Verification items for the finished model (mm, model axes). Face numbers are marked on the shaded views. A direction names the side the tool comes from. Coordinates: 2 decimals unless noted, no trailing zeros. Write each loop counter-clockwise with the first axis right and the second up, starting at its lowest first coordinate (ties: lowest second). Pieces come first, ordered by that corner, then holes. Notation, with made-up numbers: (-3.5, 89) -> (30.5, 89) arc R12 cw to (30.5, 93) -> close; hole circle Ø6 at (47, -33). An arc over 180 degrees is marked (long way). Use CSV: the item, a comma, the result in double quotes.
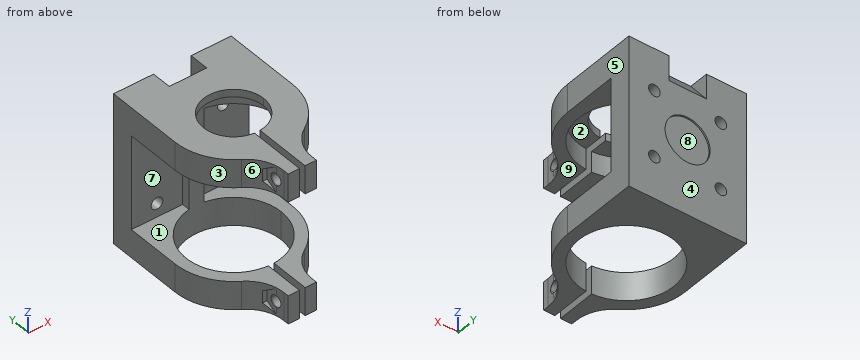
```python
from build123d import *

# Parameters (mm, degrees)
BOSS_EXTRUDE1_DEPTH   = 20
SKETCH2_W             = 3
SKETCH2_H             = 10.5
BOSS_EXTRUDE2_DEPTH   = 20
SKETCH4_W             = 31.3
SKETCH4_H             = 40
BOSS_EXTRUDE3_DEPTH   = 5
SKETCH5_W             = 25
SKETCH5_H             = 37.777747226
CUT_EXTRUDE2_DEPTH    = 13.65
SKETCH6_R             = 1.55
MOTORMOUNTHOLES_DEPTH = 6
CLAMPHOLES_REACH      = 38.211
SKETCH8_R             = 1.55
ENDSTOPPER_DEPTH      = 2
CUT_EXTRUDE7_START    = -15.65
SKETCH10_W            = 25
SKETCH10_H            = 37.777747226
CUT_EXTRUDE7_DEPTH    = 13.65
SKETCH11_W            = 25
SKETCH11_H            = 10.636850541
CUT_EXTRUDE8_DEPTH    = 4
FILLET1_START         = -20
FILLET1_DEPTH         = 2.1999999
FILLET1_START_2       = -14.6999999
FILLET1_2_DEPTH       = 2.1999999
FILLET1_START_3       = 12.5
FILLET1_3_DEPTH       = 2.1999999
FILLET1_START_4       = 17.8000001
FILLET1_4_DEPTH       = 2.1999999
FILLET1_START_5       = -17.8000001
FILLET1_5_DEPTH       = 3.1000002
FILLET1_START_6       = 14.6999999
FILLET1_6_DEPTH       = 3.1000002
FILLET1_START_7       = -8.389376218
FILLET1_7_OUTLINE_R   = 1.55
FILLET1_7_DEPTH       = 16.778752436
SKETCH13_W            = 10
SKETCH13_H            = 10
CUT_EXTRUDE10_REACH   = 40.348
CUT_EXTRUDE10_START   = 4
SKETCH15_R            = 3
CUT_EXTRUDE11_START   = -4
CUT_EXTRUDE11_DEPTH   = 3
SKETCH17_R            = 6
SHAFT_CLEARANCE_DEPTH = 0.4


with BuildPart() as part:
    # Sketch1 → Boss-Extrude1 (new, symmetric)
    with BuildSketch(Plane.XY):
        with BuildLine():
            Line((-15.65, 15.65), (-15.65, 0))
            ThreePointArc((-15.65, 0), (-11.066221106, 11.066221145), (5.4e-08, 15.65))
            Line((5.4e-08, 15.65), (-15.65, 15.65))
        make_face()
        with BuildLine():
            Line((15.65, 15.65), (5.4e-08, 15.65))
            ThreePointArc((5.4e-08, 15.65), (11.066221145, 11.066221106), (15.65, 0))
            Line((15.65, 0), (15.65, 15.65))
        make_face()
        with BuildLine():
            ThreePointArc((5.4e-08, 15.65), (-11.066221106, 11.066221145), (-15.65, 0))
            ThreePointArc((-15.65, 0), (-11.328283189, -10.797800702), (-0.75, -15.632018424))
            Line((-0.75, -15.632018424), (-0.75, -12.627747226))
            ThreePointArc((-0.75, -12.627747226), (-8.675684411, 9.206247878), (12.65, 0))
            ThreePointArc((12.65, 0), (9.206247878, -8.675684411), (0.75, -12.627747226))
            Line((0.75, -12.627747226), (0.75, -15.632018424))
            ThreePointArc((0.75, -15.632018424), (11.328283189, -10.797800702), (15.65, 0))
            ThreePointArc((15.65, 0), (11.066221145, 11.066221106), (5.4e-08, 15.65))
        make_face()
    extrude(amount=BOSS_EXTRUDE1_DEPTH, both=True)

    # Sketch2 → Boss-Extrude2 (add, symmetric)
    with BuildSketch(Plane.XY):
        with Locations((-2.25, -17.877747226)):
            Rectangle(SKETCH2_W, SKETCH2_H)
        with Locations((2.25, -17.877747226)):
            Rectangle(SKETCH2_W, SKETCH2_H)
    extrude(amount=BOSS_EXTRUDE2_DEPTH, both=True)

    # Sketch4 → Boss-Extrude3 (add)
    with BuildSketch(Plane(origin=(0, 15.65, 0), x_dir=(1, 0, 0), z_dir=(0, 1, 0))):
        Rectangle(SKETCH4_W, SKETCH4_H)
    extrude(amount=BOSS_EXTRUDE3_DEPTH)

    # Sketch5 → Cut-Extrude2 (cut)
    with BuildSketch(Plane(origin=(15.65, 0, 0), x_dir=(0, 0, -1), z_dir=(1, 0, 0))):
        with Locations((0, -4.238873613)):
            Rectangle(SKETCH5_W, SKETCH5_H)
    extrude(amount=-CUT_EXTRUDE2_DEPTH, mode=Mode.SUBTRACT)

    # Sketch6 → MotorMountHoles (cut)
    with BuildSketch(Plane(origin=(0, 20.65, 0), x_dir=(1, 0, 0), z_dir=(0, 1, 0))):
        with Locations(Location((-8.838834765, 8.838834765, 0), (0, 0, 270))):
            Circle(SKETCH6_R)
        with Locations(Location((8.838834765, 8.838834765, 0), (0, 0, 270))):
            Circle(SKETCH6_R)
        with Locations(Location((8.838834765, -8.838834765, 0), (0, 0, 270))):
            Circle(SKETCH6_R)
        with Locations(Location((-8.838834765, -8.838834765, 0), (0, 0, 270))):
            Circle(SKETCH6_R)
    extrude(amount=-MOTORMOUNTHOLES_DEPTH, mode=Mode.SUBTRACT)

    # ClampHoles: up to this face of the body (flat: up to its plane)
    clampholes_end = Plane(part.part.faces().sort_by_distance((3.75, -19.16091251, 16.25))[0])
    # Sketch8 → ClampHoles (cut, up to the picked face)
    with BuildSketch(Plane.ZY.offset(3.75), mode=Mode.PRIVATE) as clampholes_sk1:
        with Locations(Location((16.25, -19.194077794, 0), (0, 0, 270))):
            Circle(SKETCH8_R)
    clampholes_tool1 = split(extrude(clampholes_sk1.sketch, amount=-CLAMPHOLES_REACH, mode=Mode.PRIVATE), bisect_by=clampholes_end, keep=Keep.BOTH, mode=Mode.PRIVATE)
    # Sketch8 → ClampHoles (cut, up to the picked face)
    with BuildSketch(Plane.ZY.offset(3.75), mode=Mode.PRIVATE) as clampholes_sk2:
        with Locations(Location((-16.25, -19.194077794, 0), (0, 0, 270))):
            Circle(SKETCH8_R)
    clampholes_tool2 = split(extrude(clampholes_sk2.sketch, amount=-CLAMPHOLES_REACH, mode=Mode.PRIVATE), bisect_by=clampholes_end, keep=Keep.BOTH, mode=Mode.PRIVATE)
    add(clampholes_tool1.solids().sort_by(Axis((-3.75, -19.194078, 16.25), (1, 0, 0)))[0], mode=Mode.SUBTRACT)
    add(clampholes_tool2.solids().sort_by(Axis((-3.75, -19.194078, -16.25), (1, 0, 0)))[0], mode=Mode.SUBTRACT)

    # Sketch9 → EndStopper (add)
    with BuildSketch(Plane.XY.offset(20)):
        with BuildLine():
            ThreePointArc((12.65, 0), (-8.675684411, 9.206247878), (-0.75, -12.627747226))
            Line((-0.75, -12.627747226), (-0.75, -7.964766161))
            ThreePointArc((-0.75, -7.964766161), (-5.385164807, 5.916079783), (8, 0))
            ThreePointArc((8, 0), (5.916079783, -5.385164807), (0.75, -7.964766161))
            Line((0.75, -7.964766161), (0.75, -12.627747226))
            ThreePointArc((0.75, -12.627747226), (9.206247878, -8.675684411), (12.65, 0))
        make_face()
    extrude(amount=-ENDSTOPPER_DEPTH)

    # Sketch10 → Cut-Extrude7 (cut)
    with BuildSketch(Plane(origin=(0, 0, 0), x_dir=(0, 0, -1), z_dir=(1, 0, 0)).offset(CUT_EXTRUDE7_START)):
        with Locations((0, -4.238873613)):
            Rectangle(SKETCH10_W, SKETCH10_H)
    extrude(amount=CUT_EXTRUDE7_DEPTH, mode=Mode.SUBTRACT)

    # Sketch11 → Cut-Extrude8 (cut)
    with BuildSketch(Plane.ZY.offset(2)):
        with Locations((0, -17.809321955)):
            Rectangle(SKETCH11_W, SKETCH11_H)
    extrude(amount=-CUT_EXTRUDE8_DEPTH, mode=Mode.SUBTRACT)

    # Fillet1: read off the stored shape, not the designer's step
    # Fillet1 outline → Fillet1 (add)
    with BuildSketch(Plane.XY.offset(FILLET1_START)):
        with BuildLine():
            Line((3.75, -15.194077794), (3.75, -21.653175287))
            ThreePointArc((3.75, -21.653175287), (4.986261134, -16.83686123), (8.389376218, -13.211391549))
            ThreePointArc((8.389376218, -13.211391549), (6.150111782, -14.39092162), (3.75, -15.194077794))
        make_face()
        with BuildLine():
            ThreePointArc((-3.75, -15.194077794), (-6.150111782, -14.39092162), (-8.389376218, -13.21139155))
            ThreePointArc((-8.389376218, -13.21139155), (-4.986261134, -16.83686123), (-3.75, -21.653175287))
            Line((-3.75, -21.653175287), (-3.75, -15.194077794))
        make_face()
    extrude(amount=FILLET1_DEPTH)

    # Fillet1 2 outline → Fillet1 2 (add)
    with BuildSketch(Plane.XY.offset(FILLET1_START_2)):
        with BuildLine():
            Line((3.75, -15.194077794), (3.75, -21.653175287))
            ThreePointArc((3.75, -21.653175287), (4.986261134, -16.83686123), (8.389376218, -13.211391549))
            ThreePointArc((8.389376218, -13.211391549), (6.150111782, -14.39092162), (3.75, -15.194077794))
        make_face()
        with BuildLine():
            ThreePointArc((-3.75, -15.194077794), (-6.150111782, -14.39092162), (-8.389376218, -13.21139155))
            ThreePointArc((-8.389376218, -13.21139155), (-4.986261134, -16.83686123), (-3.75, -21.653175287))
            Line((-3.75, -21.653175287), (-3.75, -15.194077794))
        make_face()
    extrude(amount=FILLET1_2_DEPTH)

    # Fillet1 3 outline → Fillet1 3 (add)
    with BuildSketch(Plane.XY.offset(FILLET1_START_3)):
        with BuildLine():
            Line((3.75, -15.194077794), (3.75, -21.653175287))
            ThreePointArc((3.75, -21.653175287), (4.986261134, -16.83686123), (8.389376218, -13.211391549))
            ThreePointArc((8.389376218, -13.211391549), (6.150111782, -14.39092162), (3.75, -15.194077794))
        make_face()
        with BuildLine():
            ThreePointArc((-3.75, -15.194077794), (-6.150111782, -14.39092162), (-8.389376218, -13.21139155))
            ThreePointArc((-8.389376218, -13.21139155), (-4.986261134, -16.83686123), (-3.75, -21.653175287))
            Line((-3.75, -21.653175287), (-3.75, -15.194077794))
        make_face()
    extrude(amount=FILLET1_3_DEPTH)

    # Fillet1 4 outline → Fillet1 4 (add)
    with BuildSketch(Plane.XY.offset(FILLET1_START_4)):
        with BuildLine():
            Line((3.75, -15.194077794), (3.75, -21.653175287))
            ThreePointArc((3.75, -21.653175287), (4.986261134, -16.83686123), (8.389376218, -13.211391549))
            ThreePointArc((8.389376218, -13.211391549), (6.150111782, -14.39092162), (3.75, -15.194077794))
        make_face()
        with BuildLine():
            ThreePointArc((-3.75, -15.194077794), (-6.150111782, -14.39092162), (-8.389376218, -13.21139155))
            ThreePointArc((-8.389376218, -13.21139155), (-4.986261134, -16.83686123), (-3.75, -21.653175287))
            Line((-3.75, -21.653175287), (-3.75, -15.194077794))
        make_face()
    extrude(amount=FILLET1_4_DEPTH)

    # Fillet1 5 outline → Fillet1 5 (add)
    with BuildSketch(Plane.XY.offset(FILLET1_START_5)):
        with BuildLine():
            Line((3.75, -15.194077794), (3.75, -21.653175287))
            ThreePointArc((3.75, -21.653175287), (4.986261134, -16.83686123), (8.389376218, -13.211391549))
            ThreePointArc((8.389376218, -13.211391549), (6.150111782, -14.39092162), (3.75, -15.194077794))
        make_face()
        with BuildLine():
            ThreePointArc((-3.75, -15.194077794), (-6.150111782, -14.39092162), (-8.389376218, -13.21139155))
            ThreePointArc((-8.389376218, -13.21139155), (-4.986261134, -16.83686123), (-3.75, -21.653175287))
            Line((-3.75, -21.653175287), (-3.75, -15.194077794))
        make_face()
    extrude(amount=FILLET1_5_DEPTH)

    # Fillet1 6 outline → Fillet1 6 (add)
    with BuildSketch(Plane.XY.offset(FILLET1_START_6)):
        with BuildLine():
            Line((3.75, -15.194077794), (3.75, -21.653175287))
            ThreePointArc((3.75, -21.653175287), (4.986261134, -16.83686123), (8.389376218, -13.211391549))
            ThreePointArc((8.389376218, -13.211391549), (6.150111782, -14.39092162), (3.75, -15.194077794))
        make_face()
        with BuildLine():
            ThreePointArc((-3.75, -15.194077794), (-6.150111782, -14.39092162), (-8.389376218, -13.21139155))
            ThreePointArc((-8.389376218, -13.21139155), (-4.986261134, -16.83686123), (-3.75, -21.653175287))
            Line((-3.75, -21.653175287), (-3.75, -15.194077794))
        make_face()
    extrude(amount=FILLET1_6_DEPTH)

    # Fillet1 7 outline → Fillet1 7 (cut)
    with BuildSketch(Plane.YZ.offset(FILLET1_START_7)):
        with Locations((-19.194077794, -16.25)):
            Circle(FILLET1_7_OUTLINE_R)
        with Locations((-19.194077794, 16.25)):
            Circle(FILLET1_7_OUTLINE_R)
    extrude(amount=FILLET1_7_DEPTH, mode=Mode.SUBTRACT)

    # Cut-Sweep1: sweep along a path in Sketch12
    with BuildLine(Plane(origin=(0, 0, 0), x_dir=(0, 0, -1), z_dir=(1, 0, 0))) as cut_sweep1_path:
        Line((-2.775739564, 34.353299637), (-30.459033802, 12.328988213))
    # Sketch13 → Cut-Sweep1 (sweep, cut)
    with BuildSketch(Plane(origin=(0, 11.963370534, -15.037269505), x_dir=(-1, 0, 0), z_dir=(0, 0.6225843191548198, -0.7825527238100508))):
        with Locations((0, 29.484397462)):
            Rectangle(SKETCH13_W, SKETCH13_H)
    sweep(path=cut_sweep1_path.line, mode=Mode.SUBTRACT)

    # Sketch15 → Cut-Extrude10 (cut, up to next)
    with BuildSketch(Plane(origin=(0, 0, 0), x_dir=(0, 0, -1), z_dir=(1, 0, 0)).offset(CUT_EXTRUDE10_START), mode=Mode.PRIVATE) as cut_extrude10_sk1:
        with Locations((16.25, -19.194077794)):
            Circle(SKETCH15_R)
    cut_extrude10_tool1 = extrude(cut_extrude10_sk1.sketch, amount=CUT_EXTRUDE10_REACH, mode=Mode.PRIVATE) & part.part
    cut_extrude10 = cut_extrude10_tool1.solids().sort_by_distance((4, -19.194078, -16.25))[0]
    add(cut_extrude10, mode=Mode.SUBTRACT)

    # Sketch16 → Cut-Extrude11 (cut)
    with BuildSketch(Plane(origin=(0, 0, 0), x_dir=(0, 0, -1), z_dir=(1, 0, 0)).offset(CUT_EXTRUDE11_START)):
        Polygon((12.959103466, -19.194077794), (14.604551733, -22.044077794), (17.895448267, -22.044077794), (19.540896534, -19.194077794), (17.895448267, -16.344077794), (14.604551733, -16.344077794), align=None)
    cut_extrude11 = extrude(amount=-CUT_EXTRUDE11_DEPTH, mode=Mode.SUBTRACT)

    # Mirror1: Cut-Extrude10, Cut-Extrude11 across plane
    add(cut_extrude10.mirror(Plane.XY), mode=Mode.SUBTRACT)
    add(cut_extrude11.mirror(Plane.XY), mode=Mode.SUBTRACT)

    # Sketch17 → Shaft Clearance (cut)
    with BuildSketch(Plane(origin=(0, 20.65, 0), x_dir=(1, 0, 0), z_dir=(0, 1, 0))):
        with Locations(Location((0, 0, 0), (0, 0, 270))):
            Circle(SKETCH17_R)
    extrude(amount=-SHAFT_CLEARANCE_DEPTH, mode=Mode.SUBTRACT)


solid = part.part
```
1) Gauge pin test, flat ends, axial feed: pin 1 (0.9 mm diameter, centred on y = -18, z = -15.5, fed in from -X); pin 2 (3.5 mm diameter, centred on y = -17.5, z = 16.5, fed in from +X); pin 3 (2 mm diameter, centred on x = -7.5, y = -14, fed in from +Z); pin 4 (5 mm diameter, centred on x = -1.5, z = 0.5, fed in from +Y). Record the tip position at first contact, or that the pin passes through.
Return value:
pin 1,"x = -4"
pin 2,"x = 5.68"
pin 3,"z = 20"
pin 4,"y = 20.25"
2) Cross-section at B-B (z = 15.5). Give the number of separate pieces and of enclosed holes in the cut face, plus the area to 3 significant figures.
Return value:
separate pieces,"3"
enclosed holes,"0"
area,"545 mm2"
3) Set-up check for the marked faces 5, 6, 7, 8 and 9: record each of +Z, -Z, +X, -X, +Y, -Y from which the full face is reachable in a straight line by a thin tool's end or side.
Return value:
face 5,"+Z, -Z, +X, +Y, -Y"
face 6,"+Z, -Z, -X, -Y"
face 7,"-X, -Y"
face 8,"+Y"
face 9,"+X, -Y"
4) Scan lines: L1, parallel to Z at x = 1, y = -15.5; L2, parallel to Y at x = -3, z = 16; L3, parallel to X at y = 20.3, z = 0. Record each from-to range of solid material in increasing order.
Return value:
L1,"-20 to -12.5, 12.5 to 20"
L2,"-23.13 to -20.72, -17.66 to -12.29, 12.29 to 18.56"
L3,"-15.65 to -6, 6 to 15.65"
5) Cross-section at C-C (y = -10). Record the boundary of the cut face in (x, z), plus the area to 3 significant figures.
Return value:
outline,"(-12.04, -20) -> (-7.75, -20) -> (-7.75, -12.5) -> (-12.04, -12.5) -> close; (-12.04, 12.5) -> (-7.75, 12.5) -> (-7.75, 18) -> (-0.75, 18) -> (-0.75, 20) -> (-12.04, 20) -> close; (0.75, 18) -> (7.75, 18) -> (7.75, 12.5) -> (12.04, 12.5) -> (12.04, 20) -> (0.75, 20) -> close; (7.75, -20) -> (12.04, -20) -> (12.04, -12.5) -> (7.75, -12.5) -> close"
area,"157 mm2"
6) Cross-section at A-A (z = 0). Record the boundary of the cut face in (x, y), plus the area to 3 significant figures.
Return value:
outline,"(-15.65, 14.65) -> (-2, 14.65) -> (-2, 12.49) arc R12.65 cw to (2, 12.49) -> (2, 14.65) -> (15.65, 14.65) -> (15.65, 20.65) -> (6, 20.65) -> (6, 20.25) -> (-6, 20.25) -> (-6, 20.65) -> (-15.65, 20.65) -> close"
area,"191 mm2"
7) Cross-section at D-D (y = 17.5). Record the boundary of the cut face in (x, z), plus the area to 3 significant figures.
Return value:
outline,"(-15.65, -20) -> (15.65, -20) -> (15.65, 20) -> (5, 20) -> (5, 17.33) -> (-5, 17.33) -> (-5, 20) -> (-15.65, 20) -> close; hole circle Ø3.1 at (-8.84, -8.84); hole circle Ø3.1 at (-8.84, 8.84); hole circle Ø3.1 at (8.84, -8.84); hole circle Ø3.1 at (8.84, 8.84)"
area,"1,200 mm2"
8) Mould release check, pull along Y, two halves, no side actions. Record for the marked faces 1, 2, 3 and 4: released by +Y, released by -Y, zero draft, split by the parting line, or undercut.
Return value:
face 1,"zero draft"
face 2,"undercut"
face 3,"released by -Y"
face 4,"released by +Y"
